Read the model definition and answer for the solid it produces. Units are mm, in the model's axes. A direction names the side the tool comes from. Coordinates: 2 decimals unless noted, no trailing zeros. Write each loop counter-clockwise with the first axis right and the second up, starting at its lowest first coordinate (ties: lowest second). Pieces come first, ordered by that corner, then holes. Notation, with made-up numbers: (83.5, 66) -> (113.5, 66) arc R30 cw to (113.5, 89) -> close; hole circle Ø10 at (61.25, 27). An arc over 180 degrees is marked (long way). Write item = value, one per line. Start each with the question number.
1) For a pull along Y with two mould halves and no side action, classify faces 6 (the face through (4, 10, -1.6)), 7 (the face through (5, 10.7, 5)), 8 (the face through (4, -3.3, 3)), 9 (the face through (4, 3.2, -1)) as released by +Y, released by -Y, zero draft, split by the parting line, or undercut.
2) Section C-C (z = 5) is taken. Determine the outline of the cut face in (x, y), plus the area to 4 significant figures.
3) Section A-A (y = 3.75) is taken. Determine the outline of the cut face in (x, z).
4) A tool of negligible diameter and unlimited length cuts with its end or side. For faces 1 (the face through (2.45, 10, -1)), 2 (the face through (6.45, 2, -1)), 3 (the face through (7.406, 1.63, 5.174)), 4 (the face through (4, 1.7, -1)), 5 (the face through (4.4, 5.3, 10.5)), from which of +Z, -Z, +X, -X, +Y, -Y can it reach the whole face along a straight path? Write none if from no direction.
5) Section B-B (x = 4.45) is taken. Determine the outline of the cut face in (y, z), plus the area to 3 significant figures.
6) Find the intervals of material crossed by line 1 along Z through (x, y) = (4.45, 1.5); line 2 along Z through (x, y) = (4.45, -0.75); line 3 along X through (y, z) = (6, 8.75), in increasing order. Write a range as from..to.
7) Flat-ended cylindrical pins translate along their axes: pin 1 Ø1 at (x, y) = (1.5, 2.5) entering from -Z; pin 2 Ø1.8 at (x, z) = (5.5, -1) entering from -Y; pin 3 Ø0.8 at (y, z) = (10, -1) entering from -X. Find the tip coordinate at first contact, or state that the pin passes through.
8) Section D-D (y = 9.75) is taken. Determine the outline of the cut face in (x, z).
from build123d import *

# Parameters (mm, degrees)
F0_W     = 8.9
F0_H     = 10.9
F1_DEPTH = 3.3
F3_DEPTH = 10.7
F4_R     = 3.2
F5_DEPTH = 10
F6_W     = 4
F6_H     = 1.5
F7_DEPTH = 1.6


with BuildPart() as f1:
    # F0 (on Front) → F1 (new body)
    with BuildSketch(Plane.XZ):
        with Locations((4.45, 5.45)):
            Rectangle(F0_W, F0_H)
    extrude(amount=F1_DEPTH)

    # F2 (on face) → F3 (join)
    with BuildSketch(Plane(origin=(0, 0, 0), x_dir=(-1, 0, 0), z_dir=(0, 1, 0))):
        with BuildLine():
            Line((-8.55, 6.4), (-8.9, 6.4))
            Line((-8.9, 6.4), (-8.9, 0))
            Line((-8.9, 0), (0, 0))
            Line((0, 0), (0, 6.4))
            Line((0, 6.4), (-0.35, 6.4))
            ThreePointArc((-0.35, 6.4), (-4.45, 10.5), (-8.55, 6.4))
        make_face()
    extrude(amount=F3_DEPTH)

    # F4 (on face) → F5 (cut)
    with BuildSketch(Plane.XZ.offset(3.3)):
        with Locations((4.45, 6.4)):
            Circle(F4_R)
    extrude(amount=-F5_DEPTH, mode=Mode.SUBTRACT)

    # F6 (on face) → F7 (join)
    with BuildSketch(Plane(origin=(0, 0, 0), x_dir=(1, 0, 0), z_dir=(0, 0, -1))):
        with Locations((4.45, -2.45)):
            Rectangle(F6_W, F6_H)
        with Locations((4.45, -9.95)):
            Rectangle(F6_W, F6_H)
    extrude(amount=F7_DEPTH)


solid = f1.part
Answer key:
q1.face_6 = zero draft
q1.face_7 = released by +Y
q1.face_8 = released by -Y
q1.face_9 = undercut
q2.outline = (0, -3.3) -> (1.57, -3.3) -> (1.57, 6.7) -> (7.33, 6.7) -> (7.33, -3.3) -> (8.9, -3.3) -> (8.9, 10.7) -> (0, 10.7) -> close
q2.area = 67.05 mm^2
q3.outline = (0, 0) -> (8.9, 0) -> (8.9, 6.4) -> (8.55, 6.4) arc R4.1 ccw to (0.35, 6.4) -> (0, 6.4) -> close; hole circle Ø6.4 at (4.45, 6.4)
q4.face_1 = -Z, -X, +Y, -Y
q4.face_2 = -Z, +X, +Y, -Y
q4.face_3 = -Y
q4.face_4 = -Z, +X, -X, -Y
q4.face_5 = +Z, +Y
q5.outline = (-3.3, 0) -> (1.7, 0) -> (1.7, -1.6) -> (3.2, -1.6) -> (3.2, 0) -> (9.2, 0) -> (9.2, -1.6) -> (10.7, -1.6) -> (10.7, 10.5) -> (0, 10.5) -> (0, 10.9) -> (-3.3, 10.9) -> (-3.3, 9.6) -> (6.7, 9.6) -> (6.7, 3.2) -> (-3.3, 3.2) -> close
q5.area = 89.1 mm^2
q6.line_1 = 0..3.2, 9.6..10.5
q6.line_2 = 0..3.2, 9.6..10.9
q6.line_3 = 1.09..2.28, 6.62..7.81
q7.pin_1 = 0
q7.pin_2 = 1.7
q7.pin_3 = 2.45
q8.outline = (0, 0) -> (2.45, 0) -> (2.45, -1.6) -> (6.45, -1.6) -> (6.45, 0) -> (8.9, 0) -> (8.9, 6.4) -> (8.55, 6.4) arc R4.1 ccw to (0.35, 6.4) -> (0, 6.4) -> close
